from build123d import *

# Parameters (mm, degrees)
SKETCH_1_R          = 1.25
EXTRUDE_1_DEPTH     = 45
EXTRUDE_2_DEPTH     = 2.5
FILLET_1_R          = 2.4
CUT_EXTRUDE_1_REACH = 107.011
SKETCH_4_R          = 1.75
SKETCH_5_W          = 60
SKETCH_5_H          = 30.019734177
CUT_EXTRUDE_2_DEPTH = 100
SKETCH_7_R          = 2
CUT_EXTRUDE_3_DEPTH = 2.5
SKETCH_8_R          = 5
SKETCH_8_R_2        = 1
EXTRUDE_7_DEPTH     = 6
CUT_EXTRUDE_4_REACH = 139.511


with BuildPart() as part:
    # Эскиз1 → Бобышка-Вытянуть1 (new body)
    with BuildSketch(Plane(origin=(0, 0, 0), x_dir=(1, 0, 0), z_dir=(0, 1, 0))):
        with BuildLine():
            Line((-82.5, 32.5), (50, 32.5))
            ThreePointArc((50, 32.5), (51.767766953, 31.767766953), (52.5, 30))
            Line((52.5, 30), (52.5, -30))
            ThreePointArc((52.5, -30), (51.767766953, -31.767766953), (50, -32.5))
            Line((50, -32.5), (-82.5, -32.5))
            ThreePointArc((-82.5, -32.5), (-84.267766953, -31.767766953), (-85, -30))
            Line((-85, -30), (-85, 30))
            ThreePointArc((-85, 30), (-84.267766953, 31.767766953), (-82.5, 32.5))
        make_face()
        with Locations((-47.144457485, 27.207649218)):
            Circle(SKETCH_1_R, mode=Mode.SUBTRACT)
        with Locations((47.144457485, -27.207649218)):
            Circle(SKETCH_1_R, mode=Mode.SUBTRACT)
        with Locations((47.144457485, 27.207649218)):
            Circle(SKETCH_1_R, mode=Mode.SUBTRACT)
        with Locations((-47.144457485, -27.207649218)):
            Circle(SKETCH_1_R, mode=Mode.SUBTRACT)
        with BuildLine():
            Line((-40.944886513, 30), (40.944886513, 30))
            ThreePointArc((40.944886513, 30), (42.446070129, 29.321532349), (42.928749224, 27.74644775))
            ThreePointArc((42.928749224, 27.74644775), (44.154618836, 24.187158388), (47.726226395, 22.997655757))
            ThreePointArc((47.726226395, 22.997655757), (49.313859351, 22.524386076), (50, 21.016482364))
            Line((50, 21.016482364), (50, -21.016482364))
            ThreePointArc((50, -21.016482364), (49.313859351, -22.524386076), (47.726226395, -22.997655757))
            ThreePointArc((47.726226395, -22.997655757), (44.154618836, -24.187158388), (42.928749224, -27.74644775))
            ThreePointArc((42.928749224, -27.74644775), (42.446070129, -29.321532349), (40.944886513, -30))
            Line((40.944886513, -30), (-40.944886513, -30))
            ThreePointArc((-40.944886513, -30), (-42.446070129, -29.321532349), (-42.928749224, -27.74644775))
            ThreePointArc((-42.928749224, -27.74644775), (-44.154618836, -24.187158388), (-47.726226395, -22.997655757))
            ThreePointArc((-47.726226395, -22.997655757), (-49.313859351, -22.524386076), (-50, -21.016482364))
            Line((-50, -21.016482364), (-50, 21.016482364))
            ThreePointArc((-50, 21.016482364), (-49.313859351, 22.524386076), (-47.726226395, 22.997655757))
            ThreePointArc((-47.726226395, 22.997655757), (-44.154618836, 24.187158388), (-42.928749224, 27.74644775))
            ThreePointArc((-42.928749224, 27.74644775), (-42.446070129, 29.321532349), (-40.944886513, 30))
        make_face(mode=Mode.SUBTRACT)
        with BuildLine():
            Line((-80, 30), (-55, 30))
            ThreePointArc((-55, 30), (-53.232233047, 29.267766953), (-52.5, 27.5))
            Line((-52.5, 27.5), (-52.5, -27.5))
            ThreePointArc((-52.5, -27.5), (-53.232233047, -29.267766953), (-55, -30))
            Line((-55, -30), (-80, -30))
            ThreePointArc((-80, -30), (-81.767766953, -29.267766953), (-82.5, -27.5))
            Line((-82.5, -27.5), (-82.5, 27.5))
            ThreePointArc((-82.5, 27.5), (-81.767766953, 29.267766953), (-80, 30))
        make_face(mode=Mode.SUBTRACT)
    extrude(amount=EXTRUDE_1_DEPTH)

    # Эскиз2 → Бобышка-Вытянуть2 (add)
    with BuildSketch(Plane.XZ):
        with BuildLine():
            Line((-82.499025459, -32.487948089), (50.01119166, -32.487948089))
            ThreePointArc((50.01119166, -32.487948089), (51.778958613, -31.755715042), (52.51119166, -29.987948089))
            Line((52.51119166, -29.987948089), (52.51119166, 30.012051911))
            ThreePointArc((52.51119166, 30.012051911), (51.778958613, 31.779818864), (50.01119166, 32.512051911))
            Line((50.01119166, 32.512051911), (-82.499025459, 32.512051911))
            ThreePointArc((-82.499025459, 32.512051911), (-84.266792412, 31.779818864), (-84.999025459, 30.012051911))
            Line((-84.999025459, 30.012051911), (-84.999025459, -29.987948089))
            ThreePointArc((-84.999025459, -29.987948089), (-84.266792412, -31.755715042), (-82.499025459, -32.487948089))
        make_face()
    extrude(amount=EXTRUDE_2_DEPTH)

    # Скругление1
    fillet_1_edges = [part.edges().sort_by_distance(p)[0] for p in [
        (51.778958613, -2.5, -31.755715042),
        (52.51119166, -2.5, 0.012051911),
        (51.778958613, -2.5, 31.779818864),
        (-16.2439169, -2.5, 32.512051911),
        (-84.266792412, -2.5, 31.779818864),
        (-84.999025459, -2.5, 0.012051911),
        (-84.266792412, -2.5, -31.755715042),
        (-16.2439169, -2.5, -32.487948089),
    ]]
    fillet(fillet_1_edges, radius=FILLET_1_R)

    # Эскиз4 → Вырез-Вытянуть1 (cut, up to next)
    with BuildSketch(Plane.ZY.offset(52.5), mode=Mode.PRIVATE) as cut_extrude_1_sk1:
        with Locations((-24, 22.5)):
            Circle(SKETCH_4_R)
    cut_extrude_1_tool1 = extrude(cut_extrude_1_sk1.sketch, amount=-CUT_EXTRUDE_1_REACH, mode=Mode.PRIVATE) & part.part
    add(cut_extrude_1_tool1.solids().sort_by_distance((-52.5, 22.5, -24))[0], mode=Mode.SUBTRACT)
    # Эскиз4 → Вырез-Вытянуть1 (cut, up to next)
    with BuildSketch(Plane.ZY.offset(52.5), mode=Mode.PRIVATE) as cut_extrude_1_sk2:
        with Locations((24, 22.5)):
            Circle(SKETCH_4_R)
    cut_extrude_1_tool2 = extrude(cut_extrude_1_sk2.sketch, amount=-CUT_EXTRUDE_1_REACH, mode=Mode.PRIVATE) & part.part
    add(cut_extrude_1_tool2.solids().sort_by_distance((-52.5, 22.5, 24))[0], mode=Mode.SUBTRACT)
    # Эскиз4 → Вырез-Вытянуть1 (cut, up to next)
    with BuildSketch(Plane.ZY.offset(52.5), mode=Mode.PRIVATE) as cut_extrude_1_sk3:
        with BuildLine():
            Line((-15.25, 22.5), (-15.25, 45))
            Line((-15.25, 45), (15.25, 45))
            Line((15.25, 45), (15.25, 22.5))
            ThreePointArc((15.25, 22.5), (0, 7.25), (-15.25, 22.5))
        make_face()
    cut_extrude_1_tool3 = extrude(cut_extrude_1_sk3.sketch, amount=-CUT_EXTRUDE_1_REACH, mode=Mode.PRIVATE) & part.part
    add(cut_extrude_1_tool3.solids().sort_by_distance((-52.5, 27.593324, 0))[0], mode=Mode.SUBTRACT)
    # Эскиз4 → Вырез-Вытянуть1 (cut, up to next)
    with BuildSketch(Plane.ZY.offset(52.5), mode=Mode.PRIVATE) as cut_extrude_1_sk4:
        with BuildLine():
            Line((14.671963407, 2.845780587), (24, 2.845780587))
            ThreePointArc((24, 2.845780587), (25.400762709, 1.445017878), (24, 0.044255169))
            Line((24, 0.044255169), (14.671963407, 0.044255169))
            ThreePointArc((14.671963407, 0.044255169), (13.271200698, 1.445017878), (14.671963407, 2.845780587))
        make_face()
    cut_extrude_1_tool4 = extrude(cut_extrude_1_sk4.sketch, amount=-CUT_EXTRUDE_1_REACH, mode=Mode.PRIVATE) & part.part
    add(cut_extrude_1_tool4.solids().sort_by_distance((-52.5, 1.445018, 19.335982))[0], mode=Mode.SUBTRACT)
    # Эскиз4 → Вырез-Вытянуть1 (cut, up to next)
    with BuildSketch(Plane.ZY.offset(52.5), mode=Mode.PRIVATE) as cut_extrude_1_sk5:
        with BuildLine():
            Line((-14.671963407, 2.845780587), (-24, 2.845780587))
            ThreePointArc((-24, 2.845780587), (-25.400762709, 1.445017878), (-24, 0.044255169))
            Line((-24, 0.044255169), (-14.671963407, 0.044255169))
            ThreePointArc((-14.671963407, 0.044255169), (-13.271200698, 1.445017878), (-14.671963407, 2.845780587))
        make_face()
    cut_extrude_1_tool5 = extrude(cut_extrude_1_sk5.sketch, amount=-CUT_EXTRUDE_1_REACH, mode=Mode.PRIVATE) & part.part
    add(cut_extrude_1_tool5.solids().sort_by_distance((-52.5, 1.445018, -19.335982))[0], mode=Mode.SUBTRACT)

    # Эскиз5 → Вырез-Вытянуть2 (cut)
    with BuildSketch(Plane(origin=(-50, 0, 0), x_dir=(0, 0, -1), z_dir=(1, 0, 0))):
        with Locations((0, 15.009867089)):
            Rectangle(SKETCH_5_W, SKETCH_5_H)
    extrude(amount=CUT_EXTRUDE_2_DEPTH, mode=Mode.SUBTRACT)

    # Эскиз7 → Вырез-Вытянуть3 (cut)
    with BuildSketch(Plane(origin=(52.5, 0, 0), x_dir=(0, 0, -1), z_dir=(1, 0, 0))):
        with Locations((0, 22.5)):
            Circle(SKETCH_7_R)
    extrude(amount=-CUT_EXTRUDE_3_DEPTH, mode=Mode.SUBTRACT)

    # Эскиз8 → Бобышка-Вытянуть7 (add)
    with BuildSketch(Plane(origin=(0, 0, 0), x_dir=(1, 0, 0), z_dir=(0, 1, 0))):
        with Locations((1.091418082, 24.583435137)):
            Circle(SKETCH_8_R)
        with Locations((1.091418082, 24.583435137)):
            Circle(SKETCH_8_R_2, mode=Mode.SUBTRACT)
        with Locations((38.091418082, 24.583435137)):
            Circle(SKETCH_8_R)
        with Locations((38.091418082, 24.583435137)):
            Circle(SKETCH_8_R_2, mode=Mode.SUBTRACT)
        with Locations((38.091418082, -12.416564863)):
            Circle(SKETCH_8_R)
        with Locations((38.091418082, -12.416564863)):
            Circle(SKETCH_8_R_2, mode=Mode.SUBTRACT)
        with Locations((1.091418082, -12.416564863)):
            Circle(SKETCH_8_R)
        with Locations((1.091418082, -12.416564863)):
            Circle(SKETCH_8_R_2, mode=Mode.SUBTRACT)
    extrude(amount=EXTRUDE_7_DEPTH)

    # Эскиз10 → Вырез-Вытянуть4 (cut, up to next)
    with BuildSketch(Plane.ZY.offset(85), mode=Mode.PRIVATE) as cut_extrude_4_sk1:
        with BuildLine():
            Line((-19.25, 22.5), (-19.25, 37))
            ThreePointArc((-19.25, 37), (-21.593145751, 42.656854249), (-27.25, 45))
            Line((-27.25, 45), (27.25, 45))
            ThreePointArc((27.25, 45), (21.593145751, 42.656854249), (19.25, 37))
            Line((19.25, 37), (19.25, 22.5))
            ThreePointArc((19.25, 22.5), (0, 3.25), (-19.25, 22.5))
        make_face()
    cut_extrude_4_tool1 = extrude(cut_extrude_4_sk1.sketch, amount=-CUT_EXTRUDE_4_REACH, mode=Mode.PRIVATE) & part.part
    add(cut_extrude_4_tool1.solids().sort_by_distance((-85, 26.266593, 0))[0], mode=Mode.SUBTRACT)


solid = part.part
The model under review builds one solid part; all positions refer to its coordinate system, in mm. A direction names the side the tool comes from. Give positions to 0.01 mm unless a question says otherwise; leave off trailing zeros. Order: outer loops, then holes, each group sorted by start corner. A loop starts at its lowest first (then second) coordinate and runs counter-clockwise, first axis right, second up. Notation, with made-up numbers: M -35.75,77.5 L 20.25,77.5 A8 cw 20.25,84.5 Z; hole C 77,60.25 d5. An arc over 180 degrees is marked long. One line per question, with ' | ' between items. Start each with the question number.
1) Mouldability with a two-part tool opening along Y and no side actions: class faces 1 (the face through (-68, 0, 0)), 2 (the face through (-51.27, 23.68, 22.71)), 3 (the face through (-52.5, 7, 0)) as pulls with the +Y half, pulls with the -Y half, needs draft (parallel to the pull), parting line crosses it, or undercut.
2) For faces 4 (the face through (44.19, 37.41, 24.15)), 5 (the face through (-51.268, 7.254, 0.335)), 6 (the face through (-84, 22, 32)), 7 (the face through (1, 22, 30)), list the 3-axis set-ups (+Z, -Z, +X, -X, +Y, -Y) from which the entire face can be reached by the end or side of a thin tool; tool diameter is ignored.
3) Wall thickness on L1, parallel to X at y = 25, z = 20; L2, parallel to Y at x = -51.65, z = -24; L3, parallel to Z at x = 39.5, y = 11.5: over which ranges is each line inside the solid? List them lowest first. Write a range as from..to.
4) Clearance check with flat-ended pins moving along their axes: P1, Ø5, axis at x = 2.5, z = -23.5, coming from the +Y side; P2, Ø2, axis at x = -45.5, y = 10.5, coming from the +Z side; P3, Ø6, axis at y = 21.5, z = -7.5, coming from the +X side; P4, Ø3, axis at x = -47.14, z = -27.21, coming from the +Y side. State where each tip first meets the part, or that it passes through.
5) Consider section D-D, the plane y = 41.5. State how many separate pieces and enclosed holes the cut face has, then the cut area to 3 significant figures.
6) Consider section C-C, the plane y = 16. Give the boundary of the cut face in (x, z).
Found:
1) face 1: pulls with the +Y half | face 2: undercut | face 3: needs draft
2) face 4: +Y | face 5: -X, +Y | face 6: +Z, -X, +Y, -Y | face 7: none
3) L1: x = -85..-82.5, -52.5..-50, 50..52.5 | L2: y = -2.5..0.04, 2.85..20.75, 24.25..45 | L3: z = -32.5..-30, 30..32.5
4) P1: stops at y = 6 | P2: stops at z = 32.5 | P3: stops at x = 52.5 | P4: stops at y = 45
5) separate pieces: 1 | enclosed holes: 4 | area: 1,130 mm²
6) outline: M -85,-30 A2.5 ccw -82.5,-32.5 L 50,-32.5 A2.5 ccw 52.5,-30 L 52.5,30 A2.5 ccw 50,32.5 L -82.5,32.5 A2.5 ccw -85,30 L -85,18.12 L -82.5,18.12 L -82.5,27.5 A2.5 cw -80,30 L -55,30 A2.5 cw -52.5,27.5 L -52.5,13.8 L -50,13.8 L -50,30 L 50,30 L 50,-30 L -50,-30 L -50,-13.8 L -52.5,-13.8 L -52.5,-27.5 A2.5 cw -55,-30 L -80,-30 A2.5 cw -82.5,-27.5 L -82.5,-18.12 L -85,-18.12 Z
